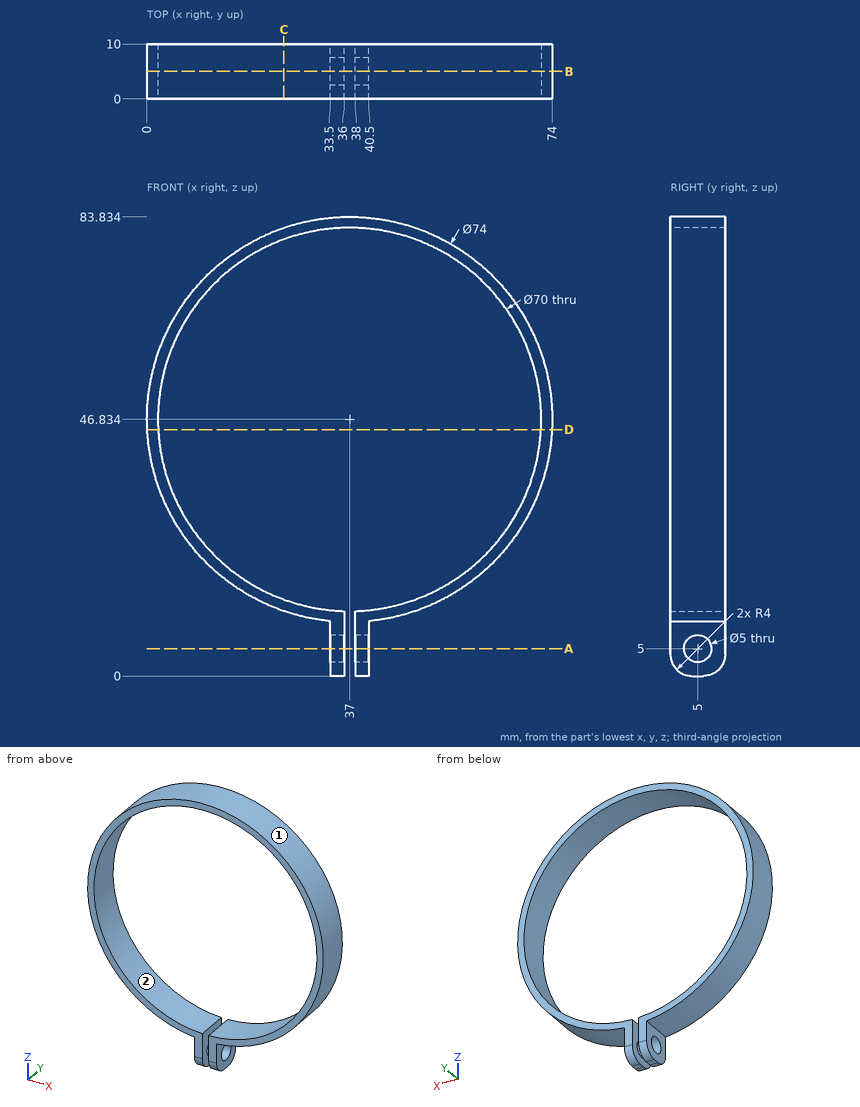
Can you work these out from the drawing? Everything is in mm from the part's minimum corner. Give positions to 0.01 mm unless a question says otherwise; leave off trailing zeros. Write each loop counter-clockwise with the first axis right and the second up, starting at its lowest first coordinate (ties: lowest second). Pieces come first, ordered by that corner, then holes. Notation, with made-up numbers: (48.25, -2) -> (83.25, -2) arc R12 cw to (83.25, 17) -> close; hole circle Ø8 at (58.25, 89.5). An arc over 180 degrees is marked (long way). Write each question's results on one line, items separated by ' | '. Start each with the question number.
Q1. We'd pull the mould along X, two halves only. Please class the marked faces 1 and 2: +X half, -X half, draft (parallel to the pull), parting line (faces both ways), or undercut.
Q2. I'm going to push flat-ended pins straight in: pin 1 Ø4 at (y, z) = (5, 5) entering from -X; pin 2 Ø3 at (y, z) = (3, 5.5) entering from -X; pin 3 Ø5 at (x, y) = (60.5, 2.5) entering from +Z; pin 4 Ø1 at (y, z) = (9, 43) entering from -X. Where does each tip first touch, or does it pass through?
Q3. Suppose I cut it at B-B, the plane y = 5. List the corners of the cut face in (x, z) for me, and give its area (3 significant figures).
Q4. Suppose I cut it at C-C, the plane x = 25. List the corners of the cut face in (y, z) for me.
Q5. Suppose I cut it at D-D, the plane z = 45. List the corners of the cut face in (x, y) for me.
Q6. Suppose I cut it at A-A, the plane z = 5. List the corners of the cut face in (x, y) for me, and give its area (3 significant figures).
Q7. I need wall thicknesses on probe 1 along X at (y, z) = (9.25, 4.5); probe 2 along Z at (x, y) = (35.5, 3); probe 3 along Y at (x, z) = (34.5, 5). Which ranges of each line are inside material? Lowest first, please.
Outcome:
1) face 1: parting line | face 2: undercut
2) pin 1: through | pin 2: x = 33.5 | pin 3: z = 77.3 | pin 4: x = 0.15
3) outline: (33.5, 0) -> (36, 0) -> (36, 2.5) -> (33.5, 2.5) -> close; (33.5, 7.5) -> (36, 7.5) -> (36, 11.85) arc R35 cw (long way) to (38, 11.85) -> (38, 7.5) -> (40.5, 7.5) -> (40.5, 10) arc R37 ccw (long way) to (33.5, 10) -> close; (38, 0) -> (40.5, 0) -> (40.5, 2.5) -> (38, 2.5) -> close | area: 473 mm2
4) outline: (0, 11.83) -> (10, 11.83) -> (10, 13.96) -> (0, 13.96) -> close; (0, 79.71) -> (10, 79.71) -> (10, 81.83) -> (0, 81.83) -> close
5) outline: (0.05, 0) -> (2.05, 0) -> (2.05, 10) -> (0.05, 10) -> close; (71.95, 0) -> (73.95, 0) -> (73.95, 10) -> (71.95, 10) -> close
6) outline: (33.5, 0) -> (36, 0) -> (36, 2.5) -> (33.5, 2.5) -> close; (33.5, 7.5) -> (36, 7.5) -> (36, 10) -> (33.5, 10) -> close; (38, 0) -> (40.5, 0) -> (40.5, 2.5) -> (38, 2.5) -> close; (38, 7.5) -> (40.5, 7.5) -> (40.5, 10) -> (38, 10) -> close | area: 25.0 mm2
7) probe 1: 33.5 to 36, 38 to 40.5 | probe 2: 0.13 to 3.5, 6.5 to 11.87, 81.8 to 83.8 | probe 3: 0 to 2.5, 7.5 to 10
